Design review of the part shown in the three views and the two pictorial views. Dimensions are in mm from the part's minimum x, y and z. A direction names the side the tool comes from. Give positions to 0.01 mm unless a question says otherwise; leave off trailing zeros. Write each loop counter-clockwise with the first axis right and the second up, starting at its lowest first coordinate (ties: lowest second). Pieces come first, ordered by that corner, then holes. Notation, with made-up numbers: M -34,19 L 22,19 A13 cw 22,27 Z; hole C 53,75.25 d2. An arc over 180 degrees is marked long. Use one line per item in the form item = value. Start each with the question number.
Q1. Consider section A-A on y = 34.5. Write out the cut boundary in (x, z).
Q2. For probe 1 along X at (y, z) = (35, 7); probe 2 along Y at (x, z) = (3.1, 6.5); probe 3 along Z at (x, y) = (1.2, 31), list the stretches that pass through material, from the lowest coordinate up. Write a range as [from, to].
Q3. Consider section B-B on z = 4.5. Write out the cut boundary in (x, y).
Q4. Clearance check with flat-ended pins moving along their axes: pin 1 Ø1.8 at (x, z) = (2.5, 4.5) entering from -Y; pin 2 Ø1 at (x, y) = (3, 17) entering from +Z. State where each tip first meets the part, or that it passes through.
Q5. Tool access review of the marked faces 1 and 2: name each direction out of +Z, -Z, +X, -X, +Y, -Y from which nothing blocks a thin tool from reaching the whole face with its end or side.
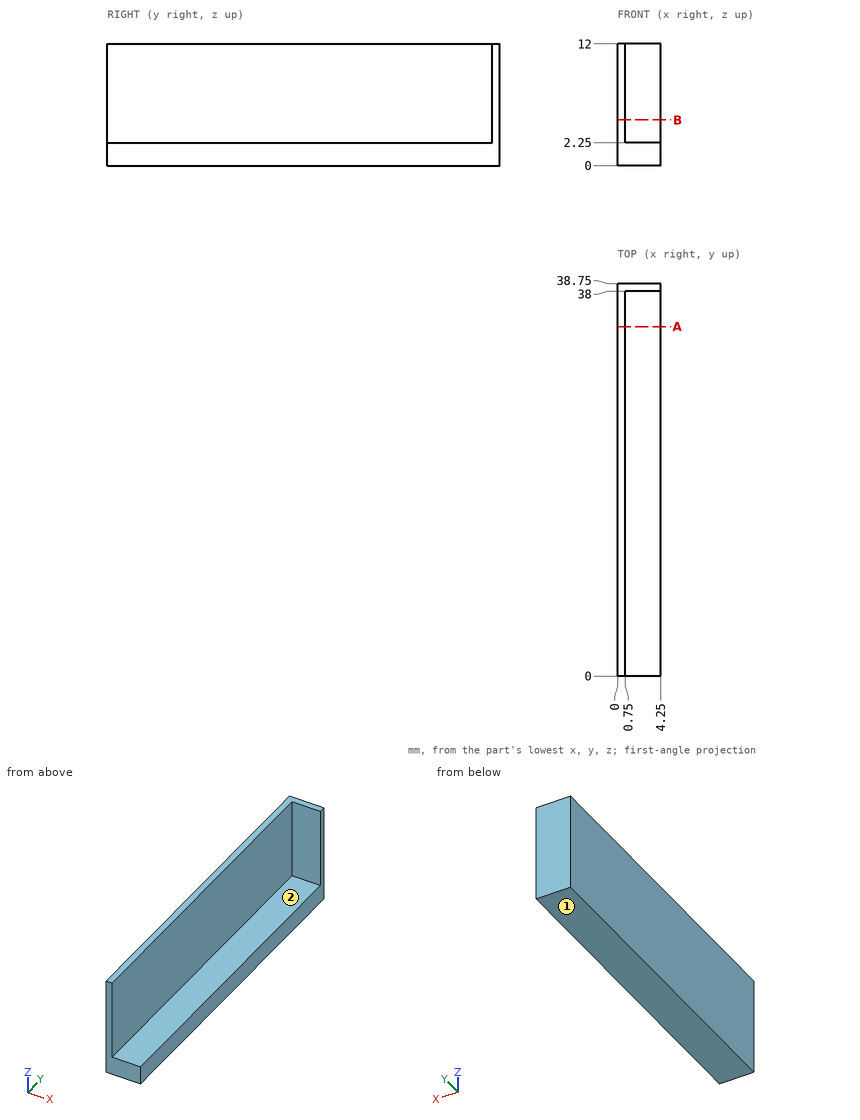
Working result:
q1.outline = M 0,0 L 4.25,0 L 4.25,2.25 L 0.75,2.25 L 0.75,12 L 0,12 Z
q2.probe_1 = [0, 0.75]
q2.probe_2 = [38, 38.75]
q2.probe_3 = [0, 2.25]
q3.outline = M 0,0 L 0.75,0 L 0.75,38 L 4.25,38 L 4.25,38.75 L 0,38.75 Z
q4.pin_1 = 38
q4.pin_2 = 2.25
q5.face_1 = -Z, +X, -X, +Y, -Y
q5.face_2 = +Z, +X, -Y
